Could you check a few things on this model? Use its own coordinates, in mm. Face numbers are marked on the shaded views. A direction names the side the tool comes from. Give positions to 0.01 mm unless a question says otherwise; leave off trailing zeros. Order: outer loops, then holes, each group sorted by start corner. A loop starts at its lowest first (then second) coordinate and runs counter-clockwise, first axis right, second up. Notation, with made-up numbers: (-15.75, 65) -> (19.25, 65) arc R26 ccw to (19.25, 88) -> close; hole circle Ø8 at (-37, 25.25). An arc over 180 degrees is marked (long way). Answer as CSV lines item,"result". Start each with the question number.
(1) Will these pins go through, and if not, where does the flat tip stop? pin 1 Ø2 at (x, y) = (10.5, 4.5) entering from -Z; pin 2 Ø3 at (x, z) = (11, 4.5) entering from +Y.
(2) I want a section at B-B (z = 3). Please give me the cut outline in (x, y), plus the area to 3 significant figures.
(3) On a 3-axis mill with a long thin cutter (end or side, diameter ignored), from which of +Z, -Z, +X, -X, +Y, -Y can I reach the whole of each face in a straight line? I mean the marked faces 1 and 2. Say none if no direction works.
(4) I need wall thicknesses on L1, parallel to X at y = 1.8, z = 3; L2, parallel to Y at x = 1.45, z = 3; L3, parallel to Y at x = 4.5, z = 1.05. Which ranges of each line are inside material? Lowest first, please.
(5) I want a section at A-A (x = 13). Please give me the cut outline in (y, z), plus the area to 3 significant figures.
(6) I want a section at D-D (y = 1.75). Please give me the cut outline in (x, z), plus the area to 3 significant figures.
(7) We'd pull the mould along Z, two halves only. Please class the marked faces 3, 4 and 5: released by +Z, released by -Z, zero draft, split by the parting line, or undercut.
```python
from build123d import *

# Parameters (mm, degrees)
EXTRUDE_1_DEPTH     = 6
SKETCH_2_R          = 1.65
CUT_EXTRUDE_1_DEPTH = 6
SKETCH_3_R          = 1.65
CUT_EXTRUDE_2_DEPTH = 6
FILLET_1_R          = 1


with BuildPart() as part:
    # 草图1 → 凸台-拉伸1 (new body)
    with BuildSketch(Plane.XY):
        Polygon((0, 0), (16, 0), (16, 3), (3, 3), (3, 12), (0, 12), align=None)
    extrude(amount=EXTRUDE_1_DEPTH)

    # 草图2 → 切除-拉伸1 (cut)
    with BuildSketch(Plane(origin=(3, 0, 0), x_dir=(0, 0, -1), z_dir=(1, 0, 0))):
        with Locations((-3, 9)):
            Circle(SKETCH_2_R)
    extrude(amount=-CUT_EXTRUDE_1_DEPTH, mode=Mode.SUBTRACT)

    # 草图3 → 切除-拉伸2 (cut)
    with BuildSketch(Plane(origin=(0, 3, 0), x_dir=(1, 0, 0), z_dir=(0, 1, 0))):
        with Locations(Location((7, -3, 0), (0, 0, 270))):
            Circle(SKETCH_3_R)
        with Locations(Location((13, -3, 0), (0, 0, 270))):
            Circle(SKETCH_3_R)
    extrude(amount=-CUT_EXTRUDE_2_DEPTH, mode=Mode.SUBTRACT)

    # 圆角1
    fillet_1_edges = [part.edges().sort_by_distance(p)[0] for p in [
        (16, 1.5, 6),
        (1.5, 12, 6),
        (1.5, 12, 0),
        (16, 1.5, 0),
    ]]
    fillet(fillet_1_edges, radius=FILLET_1_R)


solid = part.part
```
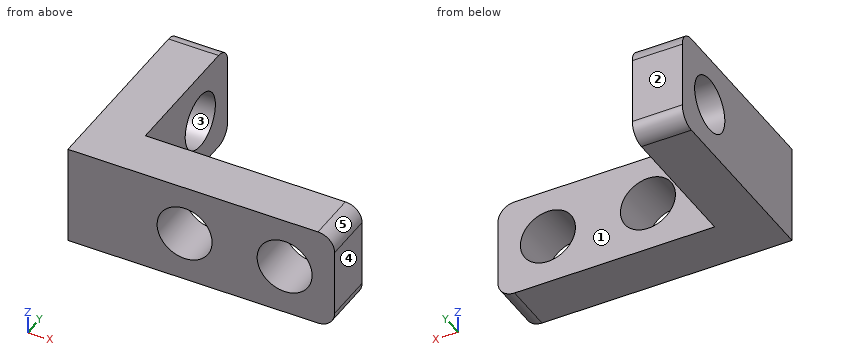
Final values:
1,pin 1,"through"
1,pin 2,"y = 3"
2,outline,"(0, 0) -> (5.35, 0) -> (5.35, 3) -> (3, 3) -> (3, 7.35) -> (0, 7.35) -> close; (0, 10.65) -> (3, 10.65) -> (3, 12) -> (0, 12) -> close; (8.65, 0) -> (11.35, 0) -> (11.35, 3) -> (8.65, 3) -> close; (14.65, 0) -> (16, 0) -> (16, 3) -> (14.65, 3) -> close"
2,area,"45.3 mm²"
3,face 1,"+Z, -Z, +X, +Y"
3,face 2,"+Z, -Z, +X, -X, +Y"
4,L1,"0 to 5.35, 8.65 to 11.35, 14.65 to 16"
4,L2,"0 to 7.35, 10.65 to 12"
4,L3,"0 to 3"
5,outline,"(0, 0) -> (3, 0) -> (3, 1.35) -> (0, 1.35) -> close; (0, 4.65) -> (3, 4.65) -> (3, 6) -> (0, 6) -> close"
5,area,"8.10 mm²"
6,outline,"(0, 0) -> (15, 0) arc R1 ccw to (16, 1) -> (16, 5) arc R1 ccw to (15, 6) -> (0, 6) -> close; hole circle Ø3.3 at (7, 3); hole circle Ø3.3 at (13, 3)"
6,area,"78.5 mm²"
7,face 3,"undercut"
7,face 4,"zero draft"
7,face 5,"released by +Z"
